Part model, mm, in its own coordinate system. A direction names the side the tool comes from. Round coordinates to 2 decimals unless told otherwise and drop trailing zeros. Write each loop counter-clockwise with the first axis right and the second up, starting at its lowest first coordinate (ties: lowest second). Pieces come first, ordered by that corner, then holes.
1) Saw through at A-A on z = -2.35. Write the cut outline in (x, y) (3 decimals).
2) Which spindle directions (+Z, -Z, +X, -X, +Y, -Y) get a long thin tool onto all of the face, cutting with end or side? Do faces 4 (the cylindrical face through (6.22, -4.936, 0.902)), 5 (the flat face through (4, 4, 1.829)), 6 (the flat face through (-6.477, 0, -2)). Say none if no direction does.
3) Saw through at D-D on z = 1.05. Write the cut outline in (x, y).
4) Saw through at B-B on y = 0. Write the cut outline in (x, z) (3 decimals).
5) Drill centre lines: L1, parallel to X at y = 0, z = -1.95 (3 decimals); L2, parallel to X at y = 4, z = 0.1. Where is each one in solid material? Low to high.
6) Pull direction Y, two halves, no side cores. Call faces 1 (the flat face through (0, 7.874, -2)), 2 (the flat face through (7.874, 0, -2)), 3 (the flat face through (0, 6.477, -2)): +Y half, -Y half, draft (parallel to the pull), parting line (faces both ways), or undercut.
```python
from build123d import *

# Parameters (mm, degrees)
F0_W     = 15.748
F0_H     = 15.748
F0_R     = 2.3749
F1_DEPTH = 3.1242
F2_DEPTH = 1.8288
F3_W     = 12.954
F3_H     = 12.954
F3_R     = 3.175
F4_DEPTH = 2.032
F3_R_2   = 2.4892
F5_DEPTH = 2.032


with BuildPart() as f1:
    # F0 (on Top) → F1 (new body)
    with BuildSketch(Plane.XY):
        Rectangle(F0_W, F0_H)
        with Locations((-4.0259, -4.0259)):
            Circle(F0_R, mode=Mode.SUBTRACT)
        with Locations((4.0259, -4.0259)):
            Circle(F0_R, mode=Mode.SUBTRACT)
        with Locations((-4.0259, 4.0259)):
            Circle(F0_R, mode=Mode.SUBTRACT)
        with Locations((4.0259, 4.0259)):
            Circle(F0_R, mode=Mode.SUBTRACT)
        with Locations((-4.0259, 4.0259)):
            Circle(F0_R)
        with Locations((-4.0259, -4.0259)):
            Circle(F0_R)
        with Locations((4.0259, -4.0259)):
            Circle(F0_R)
        with Locations((4.0259, 4.0259)):
            Circle(F0_R)
    extrude(amount=-F1_DEPTH)

    # F0 (on Top) → F2 (join)
    with BuildSketch(Plane.XY):
        with Locations((-4.0259, 4.0259)):
            Circle(F0_R)
        with Locations((-4.0259, -4.0259)):
            Circle(F0_R)
        with Locations((4.0259, -4.0259)):
            Circle(F0_R)
        with Locations((4.0259, 4.0259)):
            Circle(F0_R)
    extrude(amount=F2_DEPTH)

    # F3 (on face) → F4 (cut)
    with BuildSketch(Plane(origin=(0, 0, -3.1242), x_dir=(1, 0, 0), z_dir=(0, 0, -1))):
        Rectangle(F3_W, F3_H)
        Circle(F3_R, mode=Mode.SUBTRACT)
    extrude(amount=-F4_DEPTH, mode=Mode.SUBTRACT)

    # F3 (on face) → F5 (cut)
    with BuildSketch(Plane(origin=(0, 0, -3.1242), x_dir=(1, 0, 0), z_dir=(0, 0, -1))):
        Circle(F3_R_2)
    extrude(amount=-F5_DEPTH, mode=Mode.SUBTRACT)


solid = f1.part
```
Completed:
1. outline: (-7.874, -7.874) - (7.874, -7.874) - (7.874, 7.874) - (-7.874, 7.874) - close; circle Ø6.35 at (0, 0); hole (-6.477, -6.477) - (6.477, -6.477) - (6.477, 6.477) - (-6.477, 6.477) - close; hole circle Ø4.978 at (0, 0)
2. face 4: +Z
2. face 5: +Z, +X, -X, +Y, -Y
2. face 6: -Z
3. outline: circle Ø4.75 at (-4.03, -4.03); circle Ø4.75 at (-4.03, 4.03); circle Ø4.75 at (4.03, -4.03); circle Ø4.75 at (4.03, 4.03)
4. outline: (-7.874, -3.124) - (-6.477, -3.124) - (-6.477, -1.092) - (-3.175, -1.092) - (-3.175, -3.124) - (-2.489, -3.124) - (-2.489, -1.092) - (2.489, -1.092) - (2.489, -3.124) - (3.175, -3.124) - (3.175, -1.092) - (6.477, -1.092) - (6.477, -3.124) - (7.874, -3.124) - (7.874, 0) - (-7.874, 0) - close
5. L1: x = -7.874 to -6.477, -3.175 to -2.489, 2.489 to 3.175, 6.477 to 7.874
5. L2: x = -6.4 to -1.65, 1.65 to 6.4
6. face 1: +Y half
6. face 2: draft
6. face 3: undercut
